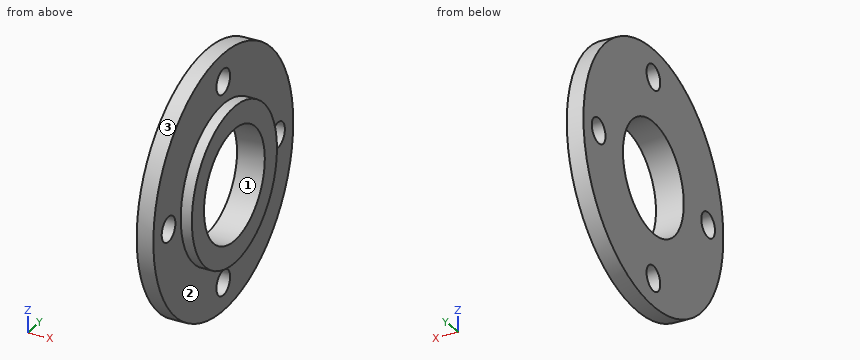
from build123d import *

# Parameters (mm, degrees)
M4_CLEARANCE_HOLE1_D     = 4.5
M4_CLEARANCE_HOLE1_DEPTH = 3
CIRPATTERN1_COUNT        = 4


with BuildPart() as part:
    # Sketch1 → Revolve1 (revolve)
    with BuildSketch(Plane.XY):
        Polygon((0, 10), (5, 10), (5, 14), (3, 14), (3, 23), (0, 23), align=None)
    revolve(axis=Axis((0, 0, 0), (1, 0, 0)))

    # M4 Clearance Hole1
    with Locations(Plane.ZY):
        with Locations((0, 18)):
            m4_clearance_hole1 = Hole(M4_CLEARANCE_HOLE1_D / 2, depth=M4_CLEARANCE_HOLE1_DEPTH)

    # CirPattern1: M4 Clearance Hole1 ×4 about axis
    cirpattern1_axis = Axis((0, 0, 0), (1, 0, 0))
    for i in range(1, CIRPATTERN1_COUNT):
        add(m4_clearance_hole1.rotate(cirpattern1_axis, i * 360 / CIRPATTERN1_COUNT), mode=Mode.SUBTRACT)


solid = part.part
Could you check a few things on this model? Use its own coordinates, in mm. Face numbers are marked on the shaded views. Give positions to 0.01 mm unless a question says otherwise; leave off trailing zeros. Order: outer loops, then holes, each group sorted by start corner. A loop starts at its lowest first (then second) coordinate and runs counter-clockwise, first axis right, second up.
1. I need wall thicknesses on L1, parallel to Z at x = 1.3, y = 0; L2, parallel to X at y = -2, z = 14; L3, parallel to Z at x = 0.85, y = -9. Which ranges of each line are inside material? Lowest first, please.
2. Suppose I cut it at D-D (y = -6.5). List the corners of the cut face in (x, z) for me.
3. Suppose I cut it at A-A (z = 7.5). List the corners of the cut face in (x, y) for me.
4. Suppose I cut it at B-B (y = 0). List the corners of the cut face in (x, z) for me.
5. We'd pull the mould along Z, two halves only. Please class the marked faces 1, 2 and 3: pulls with the +Z half, pulls with the -Z half, needs draft (parallel to the pull), parting line crosses it, or undercut.
6. Will these pins go through, and if not, where does the flat tip stop? P1, Ø14, axis at y = -8.5, z = 3.5, coming from the +X side; P2, Ø2, axis at x = 3, z = -7.5, coming from the -Y side; P3, Ø3, axis at x = 1, y = 12.5, coming from the -Z side; P4, Ø3, axis at x = 4, z = -12, coming from the -Y side.
7. Suppose I cut it at C-C (x = 1.05). List the corners of the cut face in (y, z) for me.
Solved:
1. L1: z = -23 to -20.25, -15.75 to -10, 10 to 15.75, 20.25 to 23
1. L2: x = 0 to 3
1. L3: z = -21.17 to -4.36, 4.36 to 21.17
2. outline: (0, -22.06) - (3, -22.06) - (3, -12.4) - (5, -12.4) - (5, -7.6) - (0, -7.6) - close; (0, 7.6) - (5, 7.6) - (5, 12.4) - (3, 12.4) - (3, 22.06) - (0, 22.06) - close
3. outline: (0, -21.74) - (3, -21.74) - (3, -11.82) - (5, -11.82) - (5, -6.61) - (0, -6.61) - close; (0, 6.61) - (5, 6.61) - (5, 11.82) - (3, 11.82) - (3, 21.74) - (0, 21.74) - close
4. outline: (0, -23) - (3, -23) - (3, -20.25) - (0, -20.25) - close; (0, -15.75) - (3, -15.75) - (3, -14) - (5, -14) - (5, -10) - (0, -10) - close; (0, 10) - (5, 10) - (5, 14) - (3, 14) - (3, 15.75) - (0, 15.75) - close; (0, 20.25) - (3, 20.25) - (3, 23) - (0, 23) - close
5. face 1: undercut
5. face 2: needs draft
5. face 3: parting line crosses it
6. P1: stops at x = 5
6. P2: stops at y = -22.06
6. P3: stops at z = -20.2
6. P4: stops at y = -20.26
7. outline: circle Ø46 at (0, 0); hole circle Ø4.5 at (-18, 0); hole circle Ø20 at (0, 0); hole circle Ø4.5 at (0, -18); hole circle Ø4.5 at (0, 18); hole circle Ø4.5 at (18, 0)
